The listing builds one solid part. Answer for the finished solid, in the listing's coordinates (mm). A direction names the side the tool comes from. Give positions to 0.01 mm unless a question says otherwise; leave off trailing zeros. Write each loop counter-clockwise with the first axis right and the second up, starting at its lowest first coordinate (ties: lowest second). Pieces come first, ordered by that corner, then holes. Notation, with made-up numbers: M -5,43.5 L 2,43.5 A32 ccw 2,73.5 Z; hole C 78.25,-15.75 d6. An arc over 180 degrees is marked long. Return JSON: item names as keys, results as strings.
from build123d import *

# Parameters (mm, degrees)
SKETCH_1_R                  = 2
SKETCH_1_W                  = 20
SKETCH_1_H                  = 40
EXTRUDE_1_DEPTH             = 8
EXTRUDE_2_DEPTH             = 5
HOLE_WIZARD_M31_D           = 3.15
PATTERN_LINEAR_1_COUNT      = 2
PATTERN_LINEAR_1_PITCH      = 18
PATTERN_LINEAR_1_COUNT_DIR2 = 2
PATTERN_LINEAR_1_PITCH_DIR2 = 85


with BuildPart() as part:
    # Эскиз1 → Бобышка-Вытянуть1 (new body)
    with BuildSketch(Plane(origin=(0, 0, 0), x_dir=(1, 0, 0), z_dir=(0, 1, 0))):
        with BuildLine():
            Line((-15, -45.596052461), (-15, 45.596052461))
            ThreePointArc((-15, 45.596052461), (0, 48), (15, 45.596052461))
            Line((15, 45.596052461), (15, -45.596052461))
            ThreePointArc((15, -45.596052461), (0, -48), (-15, -45.596052461))
        make_face()
        with Locations((-5, -34)):
            Circle(SKETCH_1_R, mode=Mode.SUBTRACT)
        with Locations((5, -34)):
            Circle(SKETCH_1_R, mode=Mode.SUBTRACT)
        with Locations((5, 14)):
            Circle(SKETCH_1_R, mode=Mode.SUBTRACT)
        with Locations((-5, 14)):
            Circle(SKETCH_1_R, mode=Mode.SUBTRACT)
        with Locations((0, -10)):
            Rectangle(SKETCH_1_W, SKETCH_1_H, mode=Mode.SUBTRACT)
    extrude(amount=EXTRUDE_1_DEPTH)

    # Эскиз2 → Бобышка-Вытянуть2 (add)
    with BuildSketch(Plane(origin=(0, 8, 0), x_dir=(1, 0, 0), z_dir=(0, 1, 0))):
        with BuildLine():
            Line((-15, 37.080992435), (-15, 45.596052461))
            ThreePointArc((-15, 45.596052461), (0, 48), (15, 45.596052461))
            Line((15, 45.596052461), (15, 37.080992435))
            ThreePointArc((15, 37.080992435), (0, 40), (-15, 37.080992435))
        make_face()
        with BuildLine():
            Line((-15, -37.080992435), (-15, -45.596052461))
            ThreePointArc((-15, -45.596052461), (0, -48), (15, -45.596052461))
            Line((15, -45.596052461), (15, -37.080992435))
            ThreePointArc((15, -37.080992435), (0, -40), (-15, -37.080992435))
        make_face()
    extrude(amount=EXTRUDE_2_DEPTH)

    # Сверло под метчик  спиральное M31 (through all)
    with Locations(Plane(origin=(0, 13, 0), x_dir=(1, 0, 0), z_dir=(0, 1, 0))):
        with Locations((-9, -42.5)):
            hole_wizard_m31 = Hole(HOLE_WIZARD_M31_D / 2)

    # Линейный массив1: Hole Wizard M31 2 × 2
    with Locations(*[(i * PATTERN_LINEAR_1_PITCH, 0, -j * PATTERN_LINEAR_1_PITCH_DIR2) for i in range(PATTERN_LINEAR_1_COUNT) for j in range(PATTERN_LINEAR_1_COUNT_DIR2) if (i, j) != (0, 0)]):
        add(hole_wizard_m31, mode=Mode.SUBTRACT)


solid = part.part
Item 1: Given pin 1 Ø3.5 at (x, z) = (9, 42.5) entering from -Y; pin 2 Ø4 at (x, y) = (-5, 5.5) entering from -Z; pin 3 Ø3 at (x, y) = (9, 5) entering from -Z; pin 4 Ø2.5 at (x, y) = (-2.5, 4.5) entering from +Z, each flat-ended and moving along its own axis, determine where each tip first touches the part or whether it passes through.
Geometry results:
{"pin 1": "stops at y = 0", "pin 2": "stops at z = -47.91", "pin 3": "stops at z = -47.41", "pin 4": "stops at z = 47.98"}
Item 2: Which of the six approach directions +Z, -Z, +X, -X, +Y, -Y give full straight-line access (tool end or side, diameter ignored) to faces 4 (the cylindrical face through (0, 10, 40)), 5 (the flat face through (0, 4, 30)), 6 (the cylindrical face through (0, 6, -48))?
Geometry results:
{"face 4": "+Y", "face 5": "+Y, -Y", "face 6": "-Z, +Y, -Y"}
Item 3: Find the intervals of material crossed by line 1 (X direction, y = 7.75, z = -42.5) (3 decimals); line 2 (X direction, y = 7.75, z = -5.5); line 3 (Z direction, x = -9, y = 5.25) (3 decimals), in increasing order.
Geometry results:
{"line 1": "x = -15 to -10.575, -7.425 to 7.425, 10.575 to 15", "line 2": "x = -15 to -10, 10 to 15", "line 3": "z = -47.149 to -44.075, -40.925 to -10, 30 to 40.925, 44.075 to 47.149"}
Item 4: A cutting plane is placed at B-B, the plane z = 42.5. Write down the section's boundary in (x, y) (3 decimals).
Geometry results:
{"outline": "M -15,0 L -10.575,0 L -10.575,13 L -15,13 Z; M -7.425,0 L 7.425,0 L 7.425,13 L -7.425,13 Z; M 10.575,0 L 15,0 L 15,13 L 10.575,13 Z"}
Item 5: A cutting plane is placed at D-D, the plane x = -5. Write down the section's boundary in (y, z).
Geometry results:
{"outline": "M 0,-47.74 L 13,-47.74 L 13,-39.69 L 8,-39.69 L 8,-16 L 0,-16 Z; M 0,-12 L 8,-12 L 8,-10 L 0,-10 Z; M 0,30 L 8,30 L 8,32 L 0,32 Z; M 0,36 L 8,36 L 8,39.69 L 13,39.69 L 13,47.74 L 0,47.74 Z"}
Item 6: Determine the mould class of faces 1 (the flat face through (0, 13, 44)), 2 (the cylindrical face through (0, 6, 48)), 3 (the flat face through (0, 4, -10)) for opening direction Z: +Z half, -Z half, draft (parallel to the pull), parting line (faces both ways), or undercut.
Geometry results:
{"face 1": "draft", "face 2": "+Z half", "face 3": "undercut"}
Item 7: A cutting plane is placed at A-A, the plane y = 11.5. Write down the section's boundary in (x, z) (3 decimals).
Geometry results:
{"outline": "M -15,-45.596 A48 ccw 15,-45.596 L 15,-37.081 A40 cw -15,-37.081 Z; M -15,37.081 A40 cw 15,37.081 L 15,45.596 A48 ccw -15,45.596 Z; hole C -9,-42.5 d3.15; hole C -9,42.5 d3.15; hole C 9,-42.5 d3.15; hole C 9,42.5 d3.15"}
Item 8: A cutting plane is placed at C-C, the plane y = 3. Count the separate pieces of the cut face and the enclosed holes in it, plus the area to 3 significant figures.
Geometry results:
{"separate pieces": "1", "enclosed holes": "9", "area": "1,950 mm2"}
